Source: CAD feature listing. Evaluate the final solid. Frame: model axes, mm. A direction names the side the tool comes from. Round coordinates to 2 decimals unless told otherwise and drop trailing zeros. Write each loop counter-clockwise with the first axis right and the second up, starting at its lowest first coordinate (ties: lowest second). Pieces come first, ordered by that corner, then holes.
Autodesk Inventor part; units mm, degrees
ref_plane "YZ Plane" through (0, 0, 0) normal (1, 0, 0) x (0, 1, 0)
ref_plane "XZ Plane" through (0, 0, 0) normal (0, 1, 0) x (-1, 0, 0)
ref_plane "XY Plane" through (0, 0, 0) normal (0, 0, 1) x (1, 0, 0)
sketch "Sketch1" plane through (0, 0, 0) normal (1, 0, 0) x (0, 1, 0)
  line L0 (23.7343, 15.4585) -> (23.7343, 4.0209)
  line L1 (23.7343, 4.0209) -> (33.6396, 9.7397)
  line L2 (33.6396, 9.7397) -> (23.7343, 15.4585)
  line L3 (32.268, 9.7397) -> (24.4201, 5.2087)
  line L4 (24.4201, 5.2087) -> (24.4201, 14.2706)
  line L5 (24.4201, 14.2706) -> (32.268, 9.7397)
  line L6 (33.6396, 9.7397) -> (23.7343, 4.0209)
  line L7 (33.6396, -1.698) -> (23.7343, 4.0209)
  line L8 (33.6396, 9.7397) -> (33.6396, -1.698)
  line L9 (32.9538, 8.5518) -> (25.1059, 4.0209)
  line L10 (25.1059, 4.0209) -> (32.9538, -0.5101)
  line L11 (32.9538, -0.5101) -> (32.9538, 8.5518)
  line L12 (23.7343, 4.0209) -> (23.7343, -7.4168)
  line L13 (23.7343, -7.4168) -> (33.6396, -1.698)
  line L14 (24.4201, -6.2289) -> (24.4201, 2.833)
  line L15 (24.4201, 2.833) -> (32.268, -1.698)
  line L16 (32.268, -1.698) -> (24.4201, -6.2289)
  line L17 (33.6396, -1.698) -> (33.6396, -13.1356)
  line L18 (33.6396, -13.1356) -> (23.7343, -7.4168)
  line L19 (32.9538, -11.9477) -> (32.9538, -2.8858)
  line L20 (25.1059, -7.4168) -> (32.9538, -11.9477)
  line L21 (32.9538, -2.8858) -> (25.1059, -7.4168)
  line L22 (23.7343, -7.4168) -> (23.7343, -18.8544)
  line L23 (24.4201, -17.6665) -> (24.4201, -8.6046)
  line L24 (23.7343, -18.8544) -> (33.6396, -13.1356)
  line L25 (32.268, -13.1356) -> (24.4201, -17.6665)
  line L26 (24.4201, -8.6046) -> (32.268, -13.1356)
  line L27 (33.6396, -13.1356) -> (33.6396, -24.5732)
  line L28 (32.9538, -14.3234) -> (25.1059, -18.8544)
  line L29 (25.1059, -18.8544) -> (32.9538, -23.3854)
  line L30 (33.6396, -24.5732) -> (23.7343, -18.8544)
  line L31 (32.9538, -23.3854) -> (32.9538, -14.3234)
  line L32 (23.7343, -18.8544) -> (23.7343, -30.292)
  line L33 (23.7343, -30.292) -> (33.6396, -24.5732)
  line L34 (32.268, -24.5732) -> (24.4201, -29.1042)
  line L35 (24.4201, -29.1042) -> (24.4201, -20.0422)
  line L36 (24.4201, -20.0422) -> (32.268, -24.5732)
  line L37 (23.7343, 4.0209) -> (13.8291, 9.7397)
  line L38 (13.8291, 9.7397) -> (23.7343, 15.4585)
  line L39 (15.2007, 9.7397) -> (23.0485, 5.2087)
  line L40 (23.0485, 5.2087) -> (23.0485, 14.2706)
  line L41 (23.0485, 14.2706) -> (15.2007, 9.7397)
  line L42 (23.7343, 4.0209) -> (13.8291, 9.7397)
  line L43 (13.8291, -1.698) -> (23.7343, 4.0209)
  line L44 (13.8291, 9.7397) -> (13.8291, -1.698)
  line L45 (14.5149, 8.5518) -> (22.3627, 4.0209)
  line L46 (22.3627, 4.0209) -> (14.5149, -0.5101)
  line L47 (14.5149, -0.5101) -> (14.5149, 8.5518)
  line L48 (13.8291, -1.698) -> (23.7343, 4.0209)
  line L49 (23.7343, -7.4168) -> (13.8291, -1.698)
  line L50 (23.0485, 2.833) -> (15.2007, -1.698)
  line L51 (23.0485, -6.2289) -> (23.0485, 2.833)
  line L52 (15.2007, -1.698) -> (23.0485, -6.2289)
  line L53 (13.8291, -13.1356) -> (23.7343, -7.4168)
  line L54 (15.2007, -13.1356) -> (23.0485, -17.6665)
  line L55 (23.0485, -17.6665) -> (23.0485, -8.6046)
  line L56 (23.7343, -18.8544) -> (13.8291, -13.1356)
  line L57 (23.0485, -8.6046) -> (15.2007, -13.1356)
  line L58 (23.7343, -7.4168) -> (13.8291, -1.698)
  line L59 (14.5149, -2.8858) -> (22.3627, -7.4168)
  line L60 (13.8291, -1.698) -> (13.8291, -13.1356)
  line L61 (14.5149, -11.9477) -> (14.5149, -2.8858)
  line L62 (13.8291, -13.1356) -> (23.7343, -7.4168)
  line L63 (22.3627, -7.4168) -> (14.5149, -11.9477)
  line L64 (13.8291, -24.5732) -> (23.7343, -18.8544)
  line L65 (23.0485, -29.1042) -> (23.0485, -20.0422)
  line L66 (23.7343, -30.292) -> (13.8291, -24.5732)
  line L67 (23.0485, -20.0422) -> (15.2007, -24.5732)
  line L68 (15.2007, -24.5732) -> (23.0485, -29.1042)
  line L69 (23.7343, -18.8544) -> (13.8291, -13.1356)
  line L70 (13.8291, -13.1356) -> (13.8291, -24.5732)
  line L71 (14.5149, -23.3854) -> (14.5149, -14.3234)
  line L72 (14.5149, -14.3234) -> (22.3627, -18.8544)
  line L73 (13.8291, -24.5732) -> (23.7343, -18.8544)
  line L74 (22.3627, -18.8544) -> (14.5149, -23.3854)
  line L75 (13.8291, 9.7397) -> (13.8291, 21.1773)
  line L76 (13.8291, 21.1773) -> (23.7343, 15.4585)
  line L77 (33.6396, 9.7397) -> (33.6396, 21.1773)
  line L78 (33.6396, 21.1773) -> (23.7343, 15.4585)
  line L79 (33.6396, 21.1773) -> (13.8291, 21.1773)
  line L80 (33.6396, -24.5732) -> (33.6396, -36.0108)
  line L81 (33.6396, -36.0108) -> (23.7343, -30.292)
  line L82 (13.8291, -24.5732) -> (13.8291, -36.0108)
  line L83 (13.8291, -36.0108) -> (23.7343, -30.292)
  line L84 (33.6396, -36.0108) -> (13.8291, -36.0108)
  line L85 (14.5149, 10.9275) -> (14.5149, 19.9894)
  line L86 (22.3627, 15.4585) -> (14.5149, 10.9275)
  line L87 (14.5149, 19.9894) -> (22.3627, 15.4585)
  line L88 (32.9538, 10.9275) -> (32.9538, 19.9894)
  line L89 (32.9538, 19.9894) -> (25.1059, 15.4585)
  line L90 (25.1059, 15.4585) -> (32.9538, 10.9275)
  line L91 (25.1059, -30.292) -> (32.9538, -34.823)
  line L92 (32.9538, -34.823) -> (32.9538, -25.761)
  line L93 (32.9538, -25.761) -> (25.1059, -30.292)
  line L94 (22.3627, -30.292) -> (14.5149, -34.823)
  line L95 (14.5149, -34.823) -> (14.5149, -25.761)
  line L96 (14.5149, -25.761) -> (22.3627, -30.292)
  line L97 (24.8388, 20.491) -> (30.3708, 20.491)
  line L98 (30.3708, 20.491) -> (23.7343, 16.2509)
  line L99 (23.7343, 16.2509) -> (16.3902, 20.491)
  line L100 (16.3902, 20.491) -> (24.8388, 20.491)
  line L101 (24.8388, -35.3246) -> (30.3708, -35.3246)
  line L102 (30.3708, -35.3246) -> (23.7343, -31.0844)
  line L103 (23.7343, -31.0844) -> (16.3902, -35.3246)
  line L104 (16.3902, -35.3246) -> (24.8388, -35.3246)
  dimension "d13" = 0.6858
extrude "Extrusion1" add sketch "Sketch1" along normal blind 10
sketch "Sketch2" plane through (0, 13.8291, 21.1773) normal (0, 0, 1) x (1, 0, 0)
  line L0 (0, 19.8105) -> (10, 19.8105)
  line L1 (10, 19.8105) -> (10, 9.9045)
  line L2 (10, 19.8105) -> (10, 0)
  line L3 (10, 9.9045) -> (4.9962, 9.9045)
  circle A0 centre (4.9962, 9.9045) radius 1.27
  point P0 (0, -13.8291)
  point P1 (0, 9.9053)
  dimension "d39" = 9.906
  dimension "d40" = 5.0038
  dimension "d41" = 2.54
sketch "Sketch3" plane through (0, 13.8291, -36.0108) normal (0, 0, -1) x (-1, 0, 0)
  line L0 (0, 19.8105) -> (-10, 19.8105)
  line L1 (0, 10.5911) -> (-10, 10.5911)
  line L2 (0, 19.8105) -> (-10, 19.8105)
  line L3 (0, 19.8105) -> (0, 9.9045)
  line L4 (0, 0) -> (0, 19.8105)
  circle A0 centre (-5.0038, 9.9053) radius 1.27
  point P0 (0, -13.8291)
  dimension "d44" = 9.906
  dimension "d46" = 2.54
extrude "Extrusion4" add sketch "Sketch2" along normal blind 3
extrude "Extrusion5" add sketch "Sketch3" along normal blind 3
properties part number "Arm support half scale"
Q1. Mould query, pull axis Y, two halves, no side actions, for faces 3 (the face through (5, 26, 21.177)), 4 (the face through (5.169, 22.475, -37.49)), 5 (the face through (5, 14.515, -19)). Classes: pulls with the +Y half, pulls with the -Y half, needs draft (parallel to the pull), parting line crosses it, or undercut.
Q2. Set-up query: faces 1 (the face through (5, 23.048, 10)), 2 (the face through (5, 24, 24.177)). Return all of +Z, -Z, +X, -X, +Y, -Y with unobstructed straight access to the full face (end or side cutting, diameter ignored); none if empty.
Q3. Pin query (flat end, axial travel): P1, Ø2, axis at x = 4, y = 17, coming from the -Z side; P2, Ø10, axis at y = 25, z = 4.5, coming from the -X side. Return the tip coordinate at first contact, or that it passes through.
Q4. Section query A-A, the plane z = 13. Output: boundary loops of the cut face in (x, y), and give its area (3 significant figures).
Q5. Section query B-B, the plane x = 7.25. Give the number of separate pieces and of enclosed holes in the cut face, and give its area (3 significant figures).
Q6. Line query: line 1 (Y direction, x = 5, z = 6); line 2 (Y direction, x = 6.5, z = 3); line 3 (Z direction, x = 9, y = 23.5). Output: solid intervals per line, ascending.
Filled in:
1. face 3: needs draft
1. face 4: parting line crosses it
1. face 5: undercut
2. face 1: +X, -X
2. face 2: +Z, +X, -X, +Y, -Y
3. P1: stops at z = -36.01
3. P2: stops at x = 0
4. outline: (0, 13.83) - (10, 13.83) - (10, 14.51) - (0, 14.51) - close; (0, 18.1) - (10, 18.1) - (10, 20.85) - (0, 20.85) - close; (0, 23.05) - (10, 23.05) - (10, 24.42) - (0, 24.42) - close; (0, 26.62) - (10, 26.62) - (10, 29.36) - (0, 29.36) - close; (0, 32.95) - (10, 32.95) - (10, 33.64) - (0, 33.64) - close
4. area: 82.3 mm2
5. separate pieces: 1
5. enclosed holes: 20
5. area: 434 mm2
6. line 1: y = 13.83 to 14.51, 18.93 to 21.68, 23.05 to 24.42, 25.79 to 28.53, 32.95 to 33.64
6. line 2: y = 13.83 to 14.51, 20.59 to 26.87, 32.95 to 33.64
6. line 3: z = -36.01 to -35.32, -31.22 to 16.39, 20.49 to 21.18
